Job drawing, mm, ordinate dimensions from the low corner. One solid piece. A direction names the side the tool comes from. Round coordinates to 2 decimals unless told otherwise and drop trailing zeros. Write each loop counter-clockwise with the first axis right and the second up, starting at its lowest first coordinate (ties: lowest second). Pieces come first, ordered by that corner, then holes.
1) Saw through at B-B on y = 37. Write the cut outline in (x, z).
2) Saw through at A-A on x = 6.25. Write the cut outline in (y, z).
3) Which spindle directions (+Z, -Z, +X, -X, +Y, -Y) get a long thin tool onto all of the face, cutting with end or side? Do the marked faces 1, 2 and 3. Say none if no direction does.
4) Drill centre lines: L1, parallel to Z at x = 18, y = 48.5; L2, parallel to X at y = 33, z = 82.5. Where is each one in solid material? Low to high.
5) Flat gauge pins, fed straight in: pin 1 (1.8 mm diameter, centred on x = 15, z = 83.5, fed in from +Y); pin 2 (3 mm diameter, centred on y = 36, z = 2, fed in from +X); pin 3 (6 mm diameter, centred on x = 16, y = 13.5, fed in from +Z). Where does each tip first touch, or does it go through?
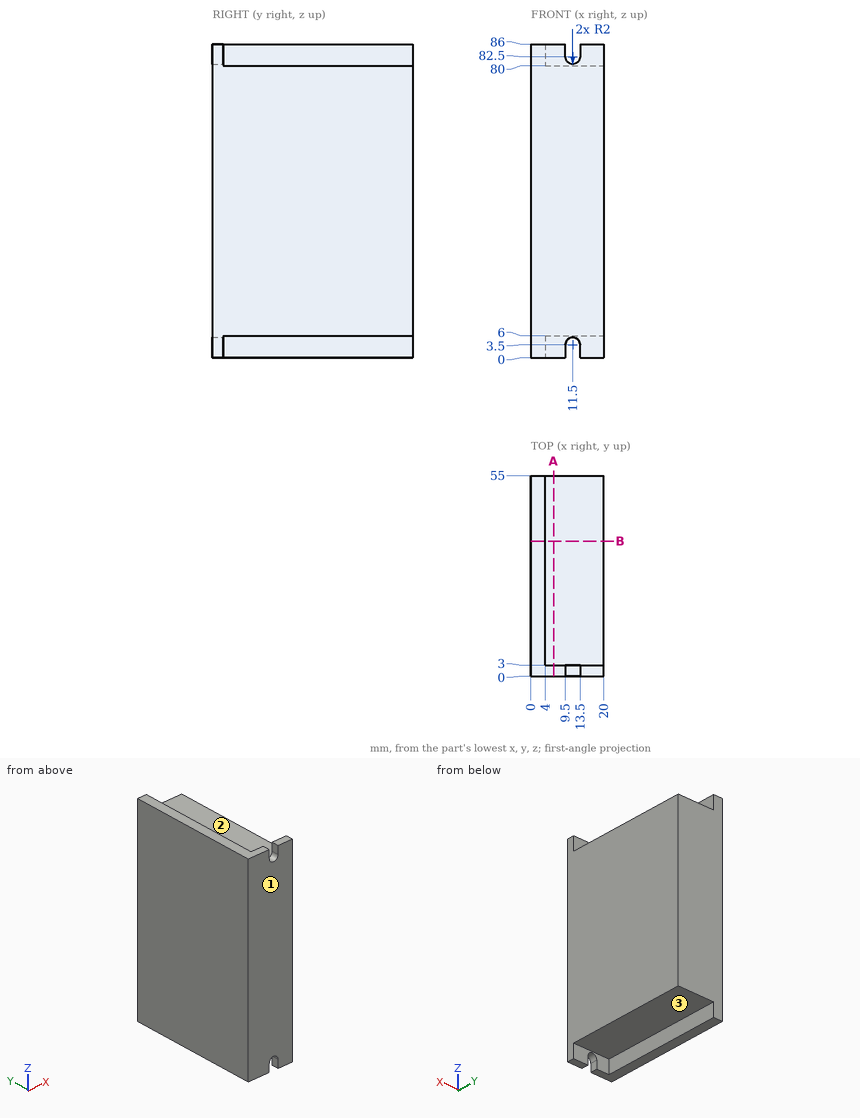
Completed:
1. outline: (0, 0) - (4, 0) - (4, 6) - (20, 6) - (20, 80) - (4, 80) - (4, 86) - (0, 86) - close
2. outline: (0, 0) - (3, 0) - (3, 6) - (55, 6) - (55, 80) - (3, 80) - (3, 86) - (0, 86) - close
3. face 1: +Z, -Z, +X, -X, -Y
3. face 2: +Z, +X, +Y
3. face 3: -Z, +X, +Y
4. L1: z = 6 to 80
4. L2: x = 0 to 4
5. pin 1: stops at y = 3
5. pin 2: stops at x = 4
5. pin 3: stops at z = 80
